```python
from build123d import *

# Parameters (mm, degrees)
ESTRUSIONE_ESTRUSIONE1_DEPTH = 506
SCHIZZO3_R                   = 2.25
TAGLIO_ESTRUSIONE1_DEPTH     = 515.719341001
SMUSSO1_SIZE                 = 1
SCHIZZO4_R                   = 2.25
TAGLIO_ESTRUSIONE2_DEPTH     = 515.719341001
SCHIZZO5_R                   = 2.25
TAGLIO_ESTRUSIONE3_DEPTH     = 515.719341001
SMUSSO2_SIZE                 = 1


with BuildPart() as part:
    # Schizzo1 → Estrusione-Estrusione1 (new body)
    with BuildSketch(Plane.XY):
        Polygon((75, 5), (75, 50), (80, 50), (80, 0), (0, 0), (0, 50), (5, 50), (5, 5), align=None)
    extrude(amount=-ESTRUSIONE_ESTRUSIONE1_DEPTH)

    # Schizzo3 → Taglio-Estrusione1 (cut, through all)
    with BuildSketch(Plane(origin=(80, 0, 0), x_dir=(0, 0, -1), z_dir=(1, 0, 0))):
        with Locations((5, 25)):
            Circle(SCHIZZO3_R)
        with Locations(Location((501, 25, 0), (0, 0, 180))):
            Circle(SCHIZZO3_R)
    extrude(amount=-TAGLIO_ESTRUSIONE1_DEPTH, mode=Mode.SUBTRACT)

    # Smusso1
    smusso1_edges = [part.edges().sort_by_distance(p)[0] for p in [
        (0, 25, -2.75),
        (80, 25, -2.75),
        (0, 25, -503.25),
        (80, 25, -503.25),
    ]]
    chamfer(smusso1_edges, length=SMUSSO1_SIZE)

    # Schizzo4 → Taglio-Estrusione2 (cut, through all)
    with BuildSketch(Plane.XZ):
        with Locations(Location((63, -253, 0), (0, 0, 270))):
            Circle(SCHIZZO4_R)
        with Locations(Location((63, -193, 0), (0, 0, 270))):
            Circle(SCHIZZO4_R)
        with Locations(Location((63, -133, 0), (0, 0, 270))):
            Circle(SCHIZZO4_R)
        with Locations(Location((63, -73, 0), (0, 0, 270))):
            Circle(SCHIZZO4_R)
        with Locations(Location((63, -13, 0), (0, 0, 270))):
            Circle(SCHIZZO4_R)
        with Locations(Location((63, -493, 0), (0, 0, 90))):
            Circle(SCHIZZO4_R)
        with Locations(Location((63, -433, 0), (0, 0, 90))):
            Circle(SCHIZZO4_R)
        with Locations(Location((63, -373, 0), (0, 0, 90))):
            Circle(SCHIZZO4_R)
        with Locations(Location((63, -313, 0), (0, 0, 90))):
            Circle(SCHIZZO4_R)
        with Locations(Location((17, -313, 0), (0, 0, 270))):
            Circle(SCHIZZO4_R)
        with Locations(Location((17, -373, 0), (0, 0, 270))):
            Circle(SCHIZZO4_R)
        with Locations(Location((17, -433, 0), (0, 0, 270))):
            Circle(SCHIZZO4_R)
        with Locations(Location((17, -493, 0), (0, 0, 270))):
            Circle(SCHIZZO4_R)
        with Locations(Location((17, -13, 0), (0, 0, 90))):
            Circle(SCHIZZO4_R)
        with Locations(Location((17, -73, 0), (0, 0, 90))):
            Circle(SCHIZZO4_R)
        with Locations(Location((17, -133, 0), (0, 0, 90))):
            Circle(SCHIZZO4_R)
        with Locations(Location((17, -193, 0), (0, 0, 90))):
            Circle(SCHIZZO4_R)
        with Locations(Location((17, -253, 0), (0, 0, 90))):
            Circle(SCHIZZO4_R)
    extrude(amount=-TAGLIO_ESTRUSIONE2_DEPTH, mode=Mode.SUBTRACT)

    # Schizzo5 → Taglio-Estrusione3 (cut, through all)
    with BuildSketch(Plane.XZ):
        with Locations(Location((26.7, -5, 0), (0, 0, 270))):
            Circle(SCHIZZO5_R)
        with Locations(Location((53.3, -5, 0), (0, 0, 270))):
            Circle(SCHIZZO5_R)
        with Locations(Location((53.3, -501, 0), (0, 0, 90))):
            Circle(SCHIZZO5_R)
        with Locations(Location((26.7, -501, 0), (0, 0, 90))):
            Circle(SCHIZZO5_R)
    extrude(amount=-TAGLIO_ESTRUSIONE3_DEPTH, mode=Mode.SUBTRACT)

    # Smusso2
    smusso2_edges = [part.edges().sort_by_distance(p)[0] for p in [
        (26.7, 0, -2.75),
        (53.3, 0, -2.75),
        (53.3, 0, -503.25),
        (26.7, 0, -503.25),
    ]]
    chamfer(smusso2_edges, length=SMUSSO2_SIZE)


solid = part.part
```
For this review, take the finished solid that the model builds, in its own axes (mm). A direction names the side the tool comes from. Coordinates: 2 decimals unless noted, no trailing zeros. Order: outer loops, then holes, each group sorted by start corner. A loop starts at its lowest first (then second) coordinate and runs counter-clockwise, first axis right, second up. Notation, with made-up numbers: (58.25, 64) - (72.25, 64) arc R18 ccw to (72.25, 85) - close; hole circle Ø2 at (-0.5, 86). An arc over 180 degrees is marked (long way). Answer as a JSON object with one key per item and string values. Group by question number.
1. We need section B-B on z = -357.5. State the section outline as (x, y) points.
2. We need section A-A on y = 36.5. State the section outline as (x, z) points, then the cut area to 3 significant figures.
3. We need section C-C on x = 10.5. State the section outline as (y, z) points, then the cut area to 3 significant figures.
4. For probe 1 along X at (y, z) = (3.9, -73); probe 2 along X at (y, z) = (3.3, -501); probe 3 along X at (y, z) = (34.5, -420.5), list the stretches that pass through material, from the lowest coordinate up.
5. Clearance check with flat-ended pins moving along their axes: P1, Ø4, axis at x = 17, z = -73, coming from the -Y side; P2, Ø5, axis at x = 63, z = -433, coming from the -Y side; P3, Ø6, axis at x = 63, z = -13, coming from the +Y side; P4, Ø6, axis at y = 25, z = -501, coming from the +X side. State where each tip first meets the part, or that it passes through.
6. The part is to be moulded in two halves that separate along X. For faces 1 (the flat face through (37.2, 4.7, -506)), 2 (the flat face through (80, 25, -249)), 3 (the flat face through (5, 28, -249)), say which applies: pulls with the +X half, pulls with the -X half, needs draft (parallel to the pull), parting line crosses it, or undercut.
7. For faces 4 (the flat face through (0, 25, -249)), 5 (the flat face through (40, 5, -249)), list the 3-axis set-ups (+Z, -Z, +X, -X, +Y, -Y) from which the entire face can be reached by the end or side of a thin tool; tool diameter is ignored.
Final values:
{
 "1": {"outline": "(0, 0) - (80, 0) - (80, 50) - (75, 50) - (75, 5) - (5, 5) - (5, 50) - (0, 50) - close"},
 "2": {"outline": "(0, -506) - (5, -506) - (5, 0) - (0, 0) - close; (75, -506) - (80, -506) - (80, 0) - (75, 0) - close", "area": "5,060 mm²"},
 "3": {"outline": "(0, -506) - (5, -506) - (5, 0) - (0, 0) - close", "area": "2,530 mm²"},
 "4": {"probe 1": "0 to 14.75, 19.25 to 60.75, 65.25 to 80", "probe 2": "0 to 24.45, 28.95 to 51.05, 55.55 to 80", "probe 3": "0 to 5, 75 to 80"},
 "5": {"P1": "through", "P2": "y = 0", "P3": "y = 5", "P4": "x = 79.75"},
 "6": {"face 1": "needs draft", "face 2": "pulls with the +X half", "face 3": "undercut"},
 "7": {"face 4": "+Z, -Z, -X, +Y, -Y", "face 5": "+Z, -Z, +Y"}
}
